from build123d import *

# Parameters (mm, degrees)
SKETCH_2_R                      = 4
CUT_EXTRUDE_2_DEPTH             = 10
CUT_EXTRUDE_4_REACH             = 42.7
CUT_EXTRUDE_4_DIRECTION_2_DEPTH = 41.70012285
CHAMFER_1_SIZE                  = 1
CUT_EXTRUDE_3_DEPTH             = 44.416471529
CUT_EXTRUDE_3_DEPTH_BACK        = 44.416471529
SKETCH_3_R                      = 1.6
SKETCH_7_R                      = 3.25
CUT_EXTRUDE_5_DEPTH             = 48.092886936
HOLE_WIZARD_M5_1_D              = 4.2


with BuildPart() as part:
    # 草图1 → 旋转1 (revolve)
    with BuildSketch(Plane.XY, mode=Mode.PRIVATE) as revolve_1_sk:
        Polygon((-5, 0), (-27.5, 0), (-27.5, 4), (-12, 4), (-12, 12), (-7, 12), (-7, 19.3), (-5, 19.3), align=None)
    revolve(revolve_1_sk.sketch.rotate(Axis((0, 0, 0), (0, 1, 0)), 270), axis=Axis((0, 0, 0), (0, 1, 0)))

    # 草图2 → 切除-拉伸2 (cut)
    with BuildSketch(Plane.XZ):
        with Locations(Location((-8.75, -15.155444566, 0), (0, 0, 270))):
            Circle(SKETCH_2_R)
        with Locations(Location((-8.75, 15.155444566, 0), (0, 0, 270))):
            Circle(SKETCH_2_R)
        with Locations(Location((8.75, 15.155444566, 0), (0, 0, 270))):
            Circle(SKETCH_2_R)
        with Locations(Location((17.5, 0, 0), (0, 0, 270))):
            Circle(SKETCH_2_R)
        with Locations(Location((8.75, -15.155444566, 0), (0, 0, 270))):
            Circle(SKETCH_2_R)
        with Locations(Location((-17.5, 0, 0), (0, 0, 270))):
            Circle(SKETCH_2_R)
    extrude(amount=-CUT_EXTRUDE_2_DEPTH, mode=Mode.SUBTRACT)

    # 切除-拉伸4: up to this face of the body (flat: up to its plane)
    cut_extrude_4_end = Plane(part.part.faces().sort_by_distance((0, 4, 26.722182541))[0])
    # 草图6 → 切除-拉伸4 (cut, up to the picked face)
    with BuildSketch(Plane.XZ.offset(-12), mode=Mode.PRIVATE) as cut_extrude_4_sk1:
        with BuildLine():
            Line((11.478240283, -3.5), (-11.478240283, -3.5))
            ThreePointArc((-11.478240283, -3.5), (0, -12), (11.478240283, -3.5))
        make_face()
    cut_extrude_4_tool1 = split(extrude(cut_extrude_4_sk1.sketch, amount=CUT_EXTRUDE_4_REACH, mode=Mode.PRIVATE), bisect_by=cut_extrude_4_end, keep=Keep.BOTH, mode=Mode.PRIVATE)
    add(cut_extrude_4_tool1.solids().sort_by(Axis((0, 12, -7.030424), (0, -1, 0)))[0], mode=Mode.SUBTRACT)

    # 草图6 → 切除-拉伸4 direction 2 (cut)
    with BuildSketch(Plane.XZ.offset(-12)):
        with BuildLine():
            Line((11.478240283, -3.5), (-11.478240283, -3.5))
            ThreePointArc((-11.478240283, -3.5), (0, -12), (11.478240283, -3.5))
        make_face()
    extrude(amount=-CUT_EXTRUDE_4_DIRECTION_2_DEPTH, mode=Mode.SUBTRACT)

    # 倒角1
    chamfer_1_edges = [part.edges().sort_by_distance(p)[0] for p in [
        (0, 12, 7),
        (0, 12, 12),
        (0, 4, 12),
        (0, 0, 5),
    ]]
    chamfer(chamfer_1_edges, length=CHAMFER_1_SIZE)

    # 草图3 → 切除-拉伸3 (cut, two sides: drawn at the far end of the back side and taken through both)
    with BuildSketch(Plane.XY.offset(-CUT_EXTRUDE_3_DEPTH_BACK)):
        with Locations((7.5, 8)):
            Circle(SKETCH_3_R)
        with Locations((-7.5, 8)):
            Circle(SKETCH_3_R)
    extrude(amount=CUT_EXTRUDE_3_DEPTH + CUT_EXTRUDE_3_DEPTH_BACK, mode=Mode.SUBTRACT)

    # 草图7 → 切除-拉伸5 (cut, through all)
    with BuildSketch(Plane(origin=(0, 0, 5.5), x_dir=(-1, 0, 0), z_dir=(0, 0, -1))):
        with Locations((-7.5, 8)):
            Circle(SKETCH_7_R)
        with Locations((7.5, 8)):
            Circle(SKETCH_7_R)
    extrude(amount=-CUT_EXTRUDE_5_DEPTH, mode=Mode.SUBTRACT)

    # M5 螺纹孔1 (through all)
    with Locations(Plane(origin=(0, 4, 0), x_dir=(1, 0, 0), z_dir=(0, 1, 0))):
        with Locations((0, 22.5), (19.485571585, 11.25), (19.485571585, -11.25), (0, -22.5), (-19.485571585, -11.25), (-19.485571585, 11.25)):
            Hole(HOLE_WIZARD_M5_1_D / 2)


solid = part.part
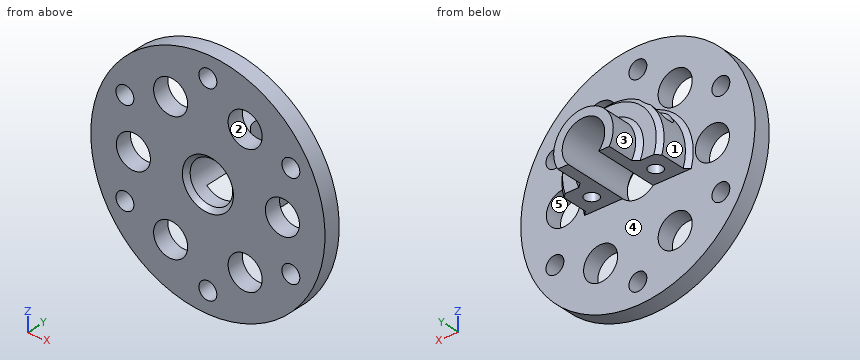
Could you check a few things on this model? Use its own coordinates, in mm. Face numbers are marked on the shaded views. A direction names the side the tool comes from. Give positions to 0.01 mm unless a question says otherwise; leave off trailing zeros. Order: outer loops, then holes, each group sorted by start corner. A loop starts at its lowest first (then second) coordinate and runs counter-clockwise, first axis right, second up.
1. I need wall thicknesses on L1, parallel to X at y = 2.95, z = 0; L2, parallel to X at y = 9.25, z = 1; L3, parallel to Y at x = 11, z = 9. Which ranges of each line are inside material? Lowest first, please.
2. Suppose I cut it at D-D (x = -24). List the corners of the cut face in (y, z) for me, plus the area to 3 significant figures.
3. Suppose I cut it at A-A (x = 0). List the corners of the cut face in (y, z) for me, plus the area to 4 significant figures.
4. We'd pull the mould along X, two halves only. Please class the marked faces 3, 4 and 5: pulls with the +X half, pulls with the -X half, needs draft (parallel to the pull), parting line crosses it, or undercut.
5. Suppose I cut it at B-B (z = -22.5). List the corners of the cut face in (x, y) for me.
6. Suppose I cut it at C-C (y = 8). List the corners of the cut face in (x, z) for me, plus the area to 3 significant figures.
7. For the marked faces 1 and 2, which set-ups out of +Z, -Z, +X, -X, +Y, -Y let a thin tool reach every point of the face, with its end or its side?
8. Will these pins go through, and if not, where does the flat tip stop? P1, Ø7, axis at x = 10, y = 15, coming from the -Z side; P2, Ø12, axis at x = -1, z = -14.5, coming from the +Y side; P3, Ø6.5, axis at x = -17.5, z = 0, coming from the -Y side; P4, Ø7, axis at x = -8, y = 9.5, coming from the +Z side.
Solved:
1. L1: x = -27.5 to -21.5, -13.5 to -5, 5 to 13.5, 21.5 to 27.5
1. L2: x = -11.96 to -8.5, -6.5 to -4.9, 4.9 to 6.5, 8.5 to 11.96
1. L3: y = 0 to 4
2. outline: (0, -13.43) - (4, -13.43) - (4, 13.43) - (0, 13.43) - close
2. area: 107 mm2
3. outline: (0, -27.5) - (4, -27.5) - (4, -24.6) - (0, -24.6) - close; (0, -20.4) - (4, -20.4) - (4, -5) - (1, -5) - (0, -6) - close; (0, 6) - (1, 5) - (19.3, 5) - (19.3, 7) - (13, 7) - (12, 8) - (12, 11) - (11, 12) - (5, 12) - (4, 13) - (4, 20.4) - (0, 20.4) - close; (0, 24.6) - (4, 24.6) - (4, 27.5) - (0, 27.5) - close
3. area: 216.5 mm2
4. face 3: parting line crosses it
4. face 4: needs draft
4. face 5: undercut
5. outline: (-15.81, 0) - (-2.1, 0) - (-2.1, 4) - (-15.81, 4) - close; (2.1, 0) - (15.81, 0) - (15.81, 4) - (2.1, 4) - close
6. outline: (-11.48, -3.5) - (-9.1, -3.5) - (-9.1, 5.5) - (-10.67, 5.5) arc R12 ccw to start; (-5.9, -3.5) - (-3.57, -3.5) arc R5 cw (long way) to (3.57, -3.5) - (5.9, -3.5) - (5.9, 5.5) - (4.25, 5.5) - (4.25, 11.22) arc R12 ccw to (-4.25, 11.22) - (-4.25, 5.5) - (-5.9, 5.5) - close; (9.1, -3.5) - (11.48, -3.5) arc R12 ccw to (10.67, 5.5) - (9.1, 5.5) - close
6. area: 134 mm2
7. face 1: -X, +Y
7. face 2: +Y, -Y
8. P1: stops at z = -3.5
8. P2: stops at y = 4
8. P3: passes through
8. P4: stops at z = 11.12
